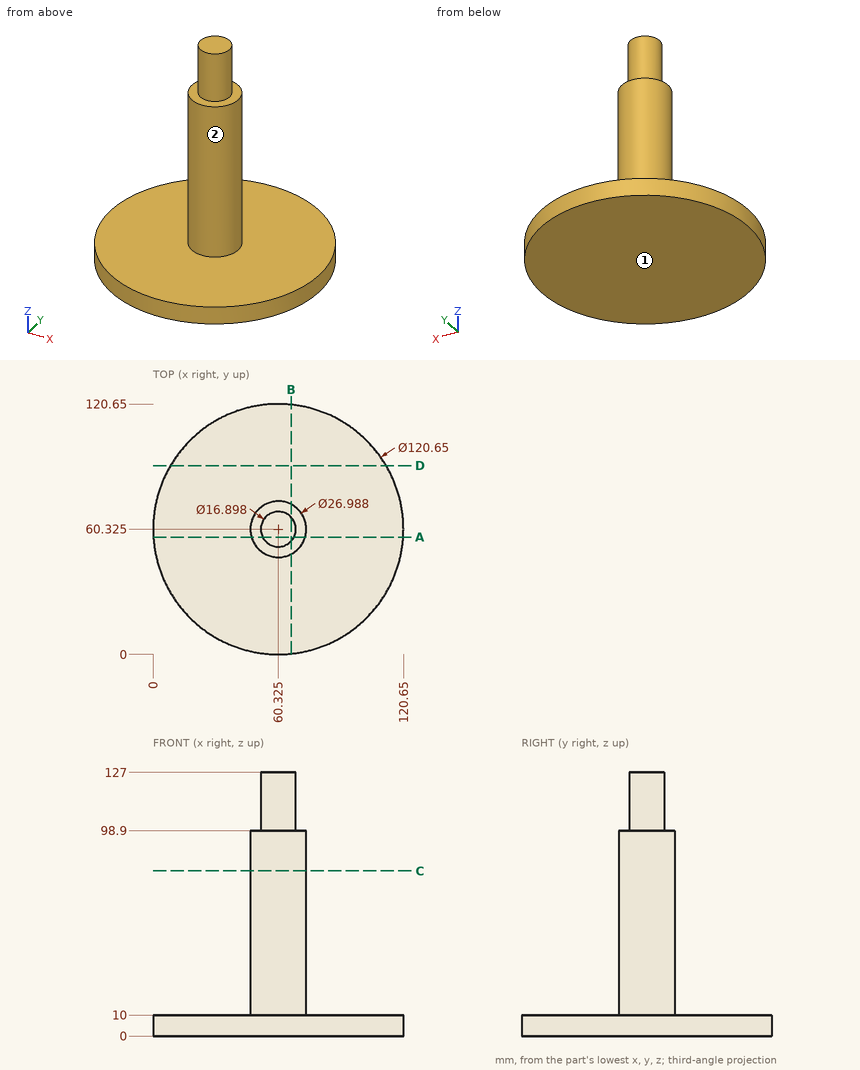
Answer from the drawing. Dimensions are ordinates in mm from the lowest x, y and z of the part. A direction names the side the tool comes from. Coordinates: 2 decimals unless noted, no trailing zeros. Loops run counter-clockwise (first coordinate to the right, second up) from the corner with the lowest first, then second, coordinate; pieces in that order, holes last. Notation, with made-up numbers: (60.25, 66.25) - (81.25, 66.25) arc R18 ccw to (81.25, 71.25) - close; hole circle Ø11 at (87, -6). An arc over 180 degrees is marked (long way). Use a Markdown table: item, result.
Item 1: Find section A-A, the plane y = 56.5. Determine the outline of the cut face in (x, z) (1 decimal), and give its area (3 significant figures).
Evaluation:
| item | result |
|---|---|
| outline | (0.1, 0) - (120.5, 0) - (120.5, 10) - (73.3, 10) - (73.3, 98.9) - (67.9, 98.9) - (67.9, 127) - (52.8, 127) - (52.8, 98.9) - (47.4, 98.9) - (47.4, 10) - (0.1, 10) - close |
| area | 3,930 mm2 |
Item 2: Given pin 1 Ø1 at (x, y) = (47.5, 62.5) entering from -Z; pin 2 Ø3 at (y, z) = (53, 36) entering from +X; pin 3 Ø12 at (y, z) = (69.5, 87) entering from +X; pin 4 Ø1.5 at (x, y) = (101.5, 83.5) entering from +Z, each flat-ended and moving along its own axis, determine where each tip first touches the part or whether it passes through.
Evaluation:
| item | result |
|---|---|
| pin 1 | stops at z = 0 |
| pin 2 | stops at x = 72.5 |
| pin 3 | stops at x = 73.44 |
| pin 4 | stops at z = 10 |
Item 3: Find section C-C, the plane z = 79.5. Determine the outline of the cut face in (x, y) (1 decimal).
Evaluation:
| item | result |
|---|---|
| outline | circle Ø27 at (60.3, 60.3) |
Item 4: Find section D-D, the plane y = 91. Determine the outline of the cut face in (x, z), and give its area (3 significant figures).
Evaluation:
| item | result |
|---|---|
| outline | (8.38, 0) - (112.27, 0) - (112.27, 10) - (8.38, 10) - close |
| area | 1,040 mm2 |
Item 5: Find section B-B, the plane x = 66.5. Determine the outline of the cut face in (y, z).
Evaluation:
| item | result |
|---|---|
| outline | (0.32, 0) - (120.33, 0) - (120.33, 10) - (72.32, 10) - (72.32, 98.9) - (66.09, 98.9) - (66.09, 127) - (54.56, 127) - (54.56, 98.9) - (48.33, 98.9) - (48.33, 10) - (0.32, 10) - close |
Item 6: Consider probe 1 along Z at (x, y) = (96, 12); probe 2 along Z at (x, y) = (54.5, 53); probe 3 along X at (y, z) = (49.5, 26.5). Determine where each line is inside the solid, lowest interval first. Write a range as from..to.
Evaluation:
| item | result |
|---|---|
| probe 1 | z = 0..10 |
| probe 2 | z = 0..98.9 |
| probe 3 | x = 52.27..68.38 |
Item 7: For the marked faces 1 and 2, determine the directions among +Z, -Z, +X, -X, +Y, -Y from which every point of the face is accessible in a straight line to the end or side of a thin tool.
Evaluation:
| item | result |
|---|---|
| face 1 | -Z, +X, -X, +Y, -Y |
| face 2 | +Z |
